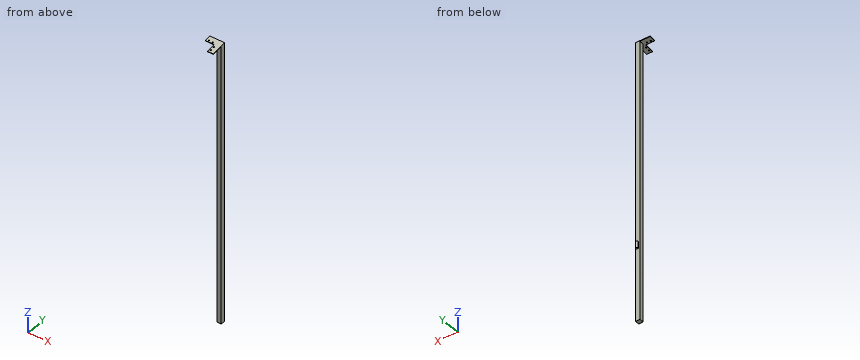
```python
from build123d import *

# Parameters (mm, degrees)
F0_W      = 45
F0_H      = 45
F1_DEPTH  = 3330
F6_W      = 45
F6_H      = 45.842251273
F7_DEPTH  = 25
F8_W      = 60
F8_H      = 60
F8_W_2    = 90
F8_H_2    = 90
F9_DEPTH  = 5
F10_R     = 6
F11_DEPTH = 25
F13_DEPTH = 5
F14_R     = 8
F15_DEPTH = 60
F16_W     = 45
F16_H     = 45
F17_DEPTH = 534
F19_DEPTH = 150.001


with BuildPart() as f1:
    # F0 (on Top) → F1 (new body)
    with BuildSketch(Plane.XY):
        Rectangle(F0_W, F0_H)
    extrude(amount=F1_DEPTH)

    # F6 (on face) → F7 (join)
    with BuildSketch(Plane(origin=(0, -624.5391596736, 3212.9754420296), x_dir=(1, 0, 0), z_dir=(0, 0.1908089954, -0.9816271834))):
        with Locations((0, -636.2284686128)):
            Rectangle(F6_W, F6_H)
    extrude(amount=F7_DEPTH)

    # F8 (on face) → F9 (join)
    with BuildSketch(Plane(origin=(0, -624.5391596736, 3212.9754420296), x_dir=(1, 0, 0), z_dir=(0, 0.1908089954, -0.9816271834))):
        with Locations((-7.5, -629.1495942493)):
            Rectangle(F8_W, F8_H)
        with Locations((-82.5, -629.1495942493)):
            Rectangle(F8_W_2, F8_H)
        with Locations((-7.5, -554.1495942493)):
            Rectangle(F8_W, F8_H_2)
    extrude(amount=F9_DEPTH)

    # F10 (on face) → F11 (cut)
    with BuildSketch(Plane(origin=(0, -624.5391596736, 3212.9754420296), x_dir=(1, 0, 0), z_dir=(0, -0.1908089954, 0.9816271834))):
        with Locations((-22.5, 534.1495942493)):
            Circle(F10_R)
        with Locations((-22.5, 574.1495942493)):
            Circle(F10_R)
        with Locations((-62.5, 614.1495942493)):
            Circle(F10_R)
        with Locations((-102.5, 614.1495942493)):
            Circle(F10_R)
    extrude(amount=-F11_DEPTH, mode=Mode.SUBTRACT)

    # F3 (on offset) → F13 (join)
    with BuildSketch(Plane.XY.offset(1256)):
        with BuildLine():
            ThreePointArc((0, 22.5), (7.0710678119, 25.4289321881), (10, 32.5))
            ThreePointArc((10, 32.5), (0, 42.5), (-10, 32.5))
            ThreePointArc((-10, 32.5), (-7.0710678119, 25.4289321881), (0, 22.5))
        make_face()
        with BuildLine():
            Line((10, 22.5), (10, 32.5))
            ThreePointArc((10, 32.5), (7.0710678119, 25.4289321881), (0, 22.5))
            Line((0, 22.5), (10, 22.5))
        make_face()
        with BuildLine():
            ThreePointArc((0, 22.5), (-7.0710678119, 25.4289321881), (-10, 32.5))
            Line((-10, 32.5), (-10, 22.5))
            Line((-10, 22.5), (0, 22.5))
        make_face()
    extrude(amount=F13_DEPTH)

    # F14 (on face) → F15 (join)
    with BuildSketch(Plane.XY.offset(1261)):
        with BuildLine():
            ThreePointArc((0, 22.5), (7.0710678119, 25.4289321881), (10, 32.5))
            ThreePointArc((10, 32.5), (0, 42.5), (-10, 32.5))
            ThreePointArc((-10, 32.5), (-7.0710678119, 25.4289321881), (0, 22.5))
        make_face()
        with Locations((0, 32.5)):
            Circle(F14_R, mode=Mode.SUBTRACT)
        with BuildLine():
            Line((10, 22.5), (10, 32.5))
            ThreePointArc((10, 32.5), (7.0710678119, 25.4289321881), (0, 22.5))
            Line((0, 22.5), (10, 22.5))
        make_face()
        with BuildLine():
            ThreePointArc((0, 22.5), (-7.0710678119, 25.4289321881), (-10, 32.5))
            Line((-10, 32.5), (-10, 22.5))
            Line((-10, 22.5), (0, 22.5))
        make_face()
    extrude(amount=F15_DEPTH)

    # F16 (on face) → F17 (cut)
    with BuildSketch(Plane(origin=(0, 0, 0), x_dir=(1, 0, 0), z_dir=(0, 0, -1))):
        Rectangle(F16_W, F16_H)
    extrude(amount=-F17_DEPTH, mode=Mode.SUBTRACT)

    # F18 (on face) → F19 (cut, through all)
    with BuildSketch(Plane.YZ.offset(22.5)):
        Polygon((22.5, 3338.7471139112), (22.5, 3313.2791965373), (27.2702248844, 3314.206434325), align=None)
    extrude(amount=-F19_DEPTH, mode=Mode.SUBTRACT)


solid = f1.part
```
The listing builds one solid part. Answer for the finished solid, in the listing's coordinates (mm). Give positions to 0.01 mm unless a question says otherwise; leave off trailing zeros. Write each loop counter-clockwise with the first axis right and the second up, starting at its lowest first coordinate (ties: lowest second). Pieces come first, ordered by that corner, then holes. Notation, with made-up numbers: (70, 15) -> (95, 15) arc R25 cw to (95, 29) -> close; hole circle Ø6 at (71, 40.5). An arc over 180 degrees is marked (long way). Use one line per item in the form item = value.
1) Each of these flat-tipped pins is pushed along its axis until it touches: P1, Ø8, axis at y = 29, z = 1288.5, coming from the +X side; P2, Ø10, axis at x = -26, y = -95, coming from the -Z side; P3, Ø13.5, axis at x = -5.5, z = 1886, coming from the -Y side. Where does it stop, or does it pass through?
Result:
P1 = 10
P2 = 3309.97
P3 = -22.5
2) Section A-A on z = 1000 is taken. Write down the section's boundary in (x, y).
Result:
outline = (-22.5, -22.5) -> (22.5, -22.5) -> (22.5, 22.5) -> (-22.5, 22.5) -> close
3) Straight lines are drawn through the part: probe 1 along Y at (x, z) = (0, 1296); probe 2 along X at (y, z) = (32, 1302); probe 3 along Y at (x, z) = (-2, 1971). For each, find the intervals that lie inside material, in ascending order.
Result:
probe_1 = -22.5 to 24.5, 40.5 to 42.5
probe_2 = -10 to -7.98, 7.98 to 10
probe_3 = -22.5 to 22.5
